Here's how the part is built. I have some questions about the finished solid (model axes, mm). Give positions to 0.01 mm unless a question says otherwise; leave off trailing zeros. Write each question's results on one line, items separated by ' | '. Start each with the question number.
Q1. I need wall thicknesses on line 1 along Y through (x, z) = (130.5, 0.6); line 2 along X through (y, z) = (12.5, 1.2); line 3 along Y through (x, z) = (-50.75, 0.75). Which ranges of each line are inside material? Lowest first, please. Write a range as [from, to].
Q2. Imagine slicing it at A-A, the plane z = 1.45. State how many separate pieces and enclosed holes the cut face has, then the cut area to 3 significant figures.
Q3. I'm going to push flat-ended pins straight in: pin 1 (3 mm diameter, centred on x = 15.18, y = -27, fed in from -Z); pin 2 (1.1 mm diameter, centred on x = 2.5, z = 1.5, fed in from +Y); pin 3 (1.1 mm diameter, centred on x = -68.5, z = 1.5, fed in from -Y). Where does each tip first touch, or does it pass through?
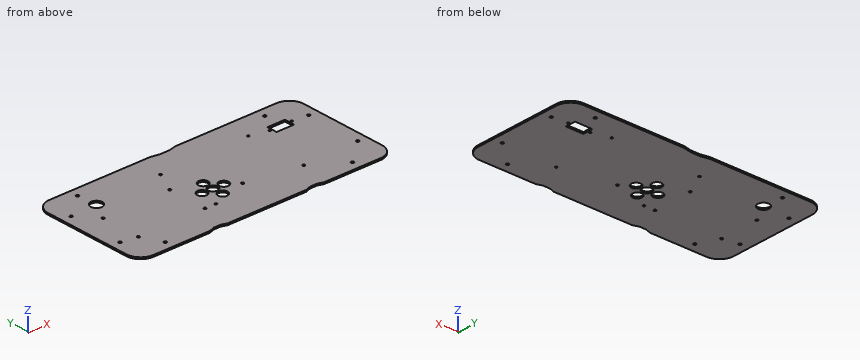
```python
from build123d import *

# Parameters (mm, degrees)
F0_R     = 1.9
F0_R_2   = 8.05
F0_R_3   = 1.475
F0_W     = 24.5
F0_H     = 14.25
F3_DEPTH = 2.286
F2_R     = 1.75
F4_DEPTH = 2.286
F1_R     = 1.55
F1_R_2   = 1.75
F1_R_3   = 6.72
F5_DEPTH = 2.286


with BuildPart() as f3:
    # F0 (on Top) → F3 (new body)
    with BuildSketch(Plane.XY):
        with BuildLine():
            Line((-17.961566, 79.945827), (-158.734, 79.945827))
            ThreePointArc((-158.734, 79.945827), (-172.922805, 74.068631), (-178.8, 59.879827))
            Line((-178.8, 59.879827), (-178.8, -61.988173))
            ThreePointArc((-178.8, -61.988173), (-172.922805, -76.176978), (-158.734, -82.054173))
            Line((-158.734, -82.054173), (-79.8, -82.054173))
            Line((-79.8, -82.054173), (-72.08434, -79.454173))
            Line((-72.08434, -79.454173), (-62.51534, -79.454173))
            Line((-62.51534, -79.454173), (-54.8, -82.054173))
            Line((-54.8, -82.054173), (54.8, -82.054173))
            Line((54.8, -82.054173), (62.515, -79.454173))
            Line((62.515, -79.454173), (72.084, -79.454173))
            Line((72.084, -79.454173), (79.8, -82.054173))
            Line((79.8, -82.054173), (158.734, -82.054173))
            ThreePointArc((158.734, -82.054173), (172.922805, -76.176978), (178.8, -61.988173))
            Line((178.8, -61.988173), (178.8, 59.879827))
            ThreePointArc((178.8, 59.879827), (172.922805, 74.068631), (158.734, 79.945827))
            Line((158.734, 79.945827), (17.961566, 79.945827))
            Line((17.961566, 79.945827), (6.5, 77.595827))
            Line((6.5, 77.595827), (-6.5, 77.595827))
            Line((-6.5, 77.595827), (-17.961566, 79.945827))
        make_face()
        with Locations((-130.9, -69.243173)):
            Circle(F0_R, mode=Mode.SUBTRACT)
        with Locations((-165.989, -38.1)):
            Circle(F0_R, mode=Mode.SUBTRACT)
        with Locations((130.9, -69.243173)):
            Circle(F0_R, mode=Mode.SUBTRACT)
        with Locations((165.989, -38.1)):
            Circle(F0_R, mode=Mode.SUBTRACT)
        with Locations((-165.989, 38.1)):
            Circle(F0_R, mode=Mode.SUBTRACT)
        with Locations((-128.8, 39.945827)):
            Circle(F0_R_2, mode=Mode.SUBTRACT)
        with Locations((-130.9, 67.134827)):
            Circle(F0_R, mode=Mode.SUBTRACT)
        with Locations((165.989, 38.1)):
            Circle(F0_R, mode=Mode.SUBTRACT)
        with Locations((113.525, 39.945827)):
            Circle(F0_R_3, mode=Mode.SUBTRACT)
        with Locations((128.8, 39.945827)):
            Rectangle(F0_W, F0_H, mode=Mode.SUBTRACT)
        with Locations((144.075, 39.95638)):
            Circle(F0_R_3, mode=Mode.SUBTRACT)
        with Locations((130.9, 67.134827)):
            Circle(F0_R, mode=Mode.SUBTRACT)
    extrude(amount=F3_DEPTH)

    # F2 (on face) → F4 (cut)
    with BuildSketch(Plane.XY):
        with Locations((-143.8, 12.895827)):
            Circle(F2_R)
        with Locations((-143.8, -42.054173)):
            Circle(F2_R)
        with Locations((-50.75, 12.895827)):
            Circle(F2_R)
        with Locations((-50.75, -42.054173)):
            Circle(F2_R)
    extrude(amount=F4_DEPTH, mode=Mode.SUBTRACT)

    # F1 (on face) → F5 (cut)
    with BuildSketch(Plane.XY):
        with Locations((88.837988, -40.262036)):
            Circle(F1_R)
        with Locations((88.837988, 46.097964)):
            Circle(F1_R)
        with Locations((-35.622012, 44.117964)):
            Circle(F1_R)
        with Locations((-35.622012, -42.242036)):
            Circle(F1_R)
        with Locations((15.177988, -27.002036)):
            Circle(F1_R_2)
        with Locations((-30.542012, -14.862036)):
            Circle(F1_R_3)
        with Locations((-15.302012, -14.862036)):
            Circle(F1_R_3)
        with Locations((-15.302012, 0.377964)):
            Circle(F1_R_3)
        with Locations((-0.062012, -14.862036)):
            Circle(F1_R_3)
        with Locations((-15.302012, -30.102036)):
            Circle(F1_R_3)
    extrude(amount=F5_DEPTH, mode=Mode.SUBTRACT)


solid = f3.part
```
Geometry check:
1) line 1: [-82.05, -71.1], [-67.39, 32.82], [47.07, 65.28], [68.99, 79.95] | line 2: [-178.8, -145.5], [-142.1, -52.45], [-49.05, 178.8] | line 3: [-82.05, -43.8], [-40.3, 11.15], [14.65, 79.95]
2) separate pieces: 1 | enclosed holes: 26 | area: 56,000 mm²
3) pin 1: through | pin 2: y = 77.6 | pin 3: y = -79.45
